```python
from build123d import *

# Parameters (mm, degrees)
SKETCH2_W            = 100
SKETCH2_H            = 80
BOSS_EXTRUDE1_DEPTH  = 50
SKETCH3_W            = 90
SKETCH3_H            = 70
CUT_EXTRUDE1_DEPTH   = 45
FILLET2_R            = 3
SKETCH4_W            = 95
SKETCH4_H            = 75
CUT_EXTRUDE2_DEPTH   = 1
SKETCH5_W            = 40
SKETCH5_H            = 10
CUT_EXTRUDE3_DEPTH   = 10
SNAP_START           = -38.217722162
SNAP_GROOVE1_DEPTH   = 3.217722162
SNAP_START_2         = -36.217722162
SNAP_GROOVE1_2_DEPTH = 1.217722162
SKETCH8_R            = 1.375
CUT_EXTRUDE4_DEPTH   = 82.240384046
LPATTERN1_COUNT      = 2
LPATTERN1_PITCH      = 58
LPATTERN1_COUNT_DIR2 = 2
LPATTERN1_PITCH_DIR2 = 49
SKETCH9_W            = 37
SKETCH9_H            = 18.5
CUT_EXTRUDE6_DEPTH   = 10


# Read off the part's stored shape, not the designer's step: Snap Groove1
with BuildPart() as part:
    # Sketch2 → Boss-Extrude1 (new body)
    with BuildSketch(Plane(origin=(0, 0, 0), x_dir=(1, 0, 0), z_dir=(0, 1, 0))):
        Rectangle(SKETCH2_W, SKETCH2_H)
    extrude(amount=BOSS_EXTRUDE1_DEPTH)

    # Sketch3 → Cut-Extrude1 (cut)
    with BuildSketch(Plane(origin=(0, 50, 0), x_dir=(1, 0, 0), z_dir=(0, 1, 0))):
        Rectangle(SKETCH3_W, SKETCH3_H)
    extrude(amount=-CUT_EXTRUDE1_DEPTH, mode=Mode.SUBTRACT)

    # Fillet2
    fillet2_edges = [part.edges().sort_by_distance(p)[0] for p in [
        (45, 27.5, -35),
        (45, 27.5, 35),
        (-45, 27.5, 35),
        (-45, 27.5, -35),
        (50, 25, 40),
        (-50, 25, 40),
        (-50, 25, -40),
        (50, 25, -40),
    ]]
    fillet(fillet2_edges, radius=FILLET2_R)

    # Sketch4 → Cut-Extrude2 (cut)
    with BuildSketch(Plane(origin=(0, 50, 0), x_dir=(1, 0, 0), z_dir=(0, 1, 0))):
        Rectangle(SKETCH4_W, SKETCH4_H)
    extrude(amount=-CUT_EXTRUDE2_DEPTH, mode=Mode.SUBTRACT)

    # Sketch5 → Cut-Extrude3 (cut)
    with BuildSketch(Plane.XY.offset(40)):
        with Locations((-22, 10)):
            Rectangle(SKETCH5_W, SKETCH5_H)
    extrude(amount=-CUT_EXTRUDE3_DEPTH, mode=Mode.SUBTRACT)

    # Snap Groove1 outline → Snap Groove1 (cut)
    with BuildSketch(Plane.XY.offset(SNAP_START)):
        Polygon((-1.245807146, 41), (0.754192854, 41), (0.911416192, 44), (-1.403030484, 44), align=None)
    snap_groove1 = extrude(amount=SNAP_GROOVE1_DEPTH, mode=Mode.SUBTRACT)

    # Snap Groove1 2 outline → Snap Groove1 2 (cut)
    with BuildSketch(Plane.XY.offset(SNAP_START_2)):
        Polygon((-1.403030484, 44), (0.911416192, 44), (1.01623175, 46), (-1.507846042, 46), align=None)
    snap_groove1_2 = extrude(amount=SNAP_GROOVE1_2_DEPTH, mode=Mode.SUBTRACT)

    # Mirror1: Snap Groove1, Snap Groove1 2 across plane
    add(snap_groove1.mirror(Plane.XY), mode=Mode.SUBTRACT)
    add(snap_groove1_2.mirror(Plane.XY), mode=Mode.SUBTRACT)

    # Sketch8 → Cut-Extrude4 (cut, through all)
    with BuildSketch(Plane.XZ):
        with Locations(Location((18.146559745, 24.040628208, 0), (0, 0, 270))):
            Circle(SKETCH8_R)
    cut_extrude4 = extrude(amount=-CUT_EXTRUDE4_DEPTH, mode=Mode.SUBTRACT)

    # LPattern1: Cut-Extrude4 2 × 2
    with Locations(*[(-i * LPATTERN1_PITCH, 0, -j * LPATTERN1_PITCH_DIR2) for i in range(LPATTERN1_COUNT) for j in range(LPATTERN1_COUNT_DIR2) if (i, j) != (0, 0)]):
        add(cut_extrude4, mode=Mode.SUBTRACT)

    # Sketch9 → Cut-Extrude6 (cut)
    with BuildSketch(Plane(origin=(50, 0, 0), x_dir=(0, 0, -1), z_dir=(1, 0, 0))):
        with Locations((-8.373367198, 14.25)):
            Rectangle(SKETCH9_W, SKETCH9_H)
    extrude(amount=-CUT_EXTRUDE6_DEPTH, mode=Mode.SUBTRACT)


solid = part.part
```
Check sheet for the modelled part. Datum: model origin and axes. Units: mm. A direction names the side the tool comes from. Give positions to 0.01 mm unless a question says otherwise; leave off trailing zeros. Loops run counter-clockwise (first coordinate to the right, second up) from the corner with the lowest first, then second, coordinate; pieces in that order, holes last. Notation, with made-up numbers: M 41.5,2.5 L 98.5,2.5 A13 ccw 98.5,19.5 Z; hole C 58,4.25 d2. An arc over 180 degrees is marked long. Answer in a Markdown table with one row per item.
1) Tool access check on faces 5 (the face through (48, 23.5, 9)), 6 (the face through (0, 43, -38.218)), 7 (the face through (-49.14, 25.35, 39.1)), 8 (the face through (-1, 27, 35)). Record the directions out of +Z, -Z, +X, -X, +Y, -Y that give a thin tool (end or side, any length) a straight path to the whole face; none if there is none.
Solutions:
| item | result |
|---|---|
| face 5 | +X |
| face 6 | none |
| face 7 | +Z, -X, +Y, -Y |
| face 8 | +Y |
2) Thickness scan on line 1 (X direction, y = 31, z = -9); line 2 (Z direction, x = -4.5, y = 41.5); line 3 (Y direction, x = -0.5, z = 15.5). Record the ranges inside material, lowest first.
Solutions:
| item | result |
|---|---|
| line 1 | x = -50 to -45, 45 to 50 |
| line 2 | z = -40 to -35, 35 to 40 |
| line 3 | y = 0 to 5 |
3) Cross-section at D-D (x = 13). Enter the section's corners in (y, z).
Solutions:
| item | result |
|---|---|
| outline | M 0,-40 L 50,-40 L 50,-37.5 L 49,-37.5 L 49,-35 L 5,-35 L 5,35 L 49,35 L 49,37.5 L 50,37.5 L 50,40 L 0,40 Z |
4) Cross-section at B-B (y = 31). Enter the section's corners in (x, z), plus the area to 3 significant figures.
Solutions:
| item | result |
|---|---|
| outline | M -50,-37 A3 ccw -47,-40 L 47,-40 A3 ccw 50,-37 L 50,37 A3 ccw 47,40 L -47,40 A3 ccw -50,37 Z; hole M -45,-32 A3 ccw -42,-35 L 42,-35 A3 ccw 45,-32 L 45,32 A3 ccw 42,35 L -42,35 A3 ccw -45,32 Z |
| area | 1,700 mm^2 |
5) Depth check by flat-ended pin: pin 1 (5 mm diameter, centred on x = 28, z = 29, fed in from +Y); pin 2 (1.6 mm diameter, centred on x = 0, z = -36, fed in from +Y); pin 3 (1.5 mm diameter, centred on x = -36.5, y = 10.5, fed in from +Z); pin 4 (2 mm diameter, centred on x = 18.15, z = 24.04, fed in from +Y). Enter the tip coordinate at first touch or a pass-through.
Solutions:
| item | result |
|---|---|
| pin 1 | stops at y = 5 |
| pin 2 | stops at y = 49 |
| pin 3 | stops at z = -35 |
| pin 4 | passes through |
6) Cross-section at C-C (x = -31.5). Enter the section's corners in (y, z), plus the area to 3 significant figures.
Solutions:
| item | result |
|---|---|
| outline | M 0,-40 L 50,-40 L 50,-37.5 L 49,-37.5 L 49,-35 L 5,-35 L 5,40 L 0,40 Z; M 15,35 L 49,35 L 49,37.5 L 50,37.5 L 50,40 L 15,40 Z |
| area | 795 mm^2 |
7) Mould release check, pull along Y, two halves, no side actions. Record for faces 1 (the face through (48, 14, 26.873)), 2 (the face through (0, 43, 38.218)), 3 (the face through (45, 32, 0)), 4 (the face through (-4, 50, 38)): released by +Y, released by -Y, zero draft, split by the parting line, or undercut.
Solutions:
| item | result |
|---|---|
| face 1 | undercut |
| face 2 | undercut |
| face 3 | zero draft |
| face 4 | released by +Y |
8) Cross-section at A-A (z = -9). Enter the section's corners in (x, y), plus the area to 4 significant figures.
Solutions:
| item | result |
|---|---|
| outline | M -50,0 L 50,0 L 50,5 L -45,5 L -45,49 L -47.5,49 L -47.5,50 L -50,50 Z; M 45,23.5 L 50,23.5 L 50,50 L 47.5,50 L 47.5,49 L 45,49 Z |
| area | 852.5 mm^2 |
